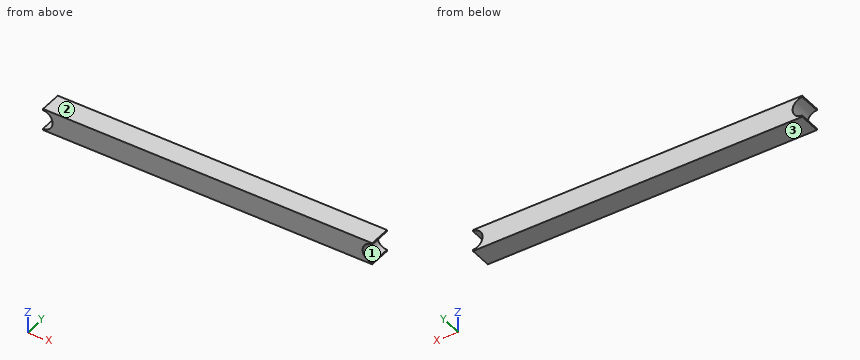
from build123d import *

# Parameters (mm, degrees)
BOX_W        = 180
BOX_H        = 12
BOX_DEPTH    = 12
POCKET_DEPTH = 12


with BuildPart() as part:
    # Box → Box (new body)
    with BuildSketch(Plane(origin=(0, -6, -6), x_dir=(1, 0, 0), z_dir=(0, 0, 1))):
        with Locations((90, 6)):
            Rectangle(BOX_W, BOX_H)
    extrude(amount=BOX_DEPTH)

    # Sketch → Pocket (cut)
    with BuildSketch(Plane(origin=(0, -6, -6), x_dir=(1, 0, 0), z_dir=(0, -1, 0))):
        with BuildLine():
            ThreePointArc((0, 0.75), (5.25, 6), (0, 11.25))
            Line((0, 11.25), (0, 0.75))
        make_face()
        with BuildLine():
            ThreePointArc((180, 11.25), (174.75, 6), (180, 0.75))
            Line((180, 11.25), (180, 0.75))
        make_face()
    extrude(amount=-POCKET_DEPTH, mode=Mode.SUBTRACT)


solid = part.part
The model under review builds one solid part; all positions refer to its coordinate system, in mm. Face numbers are marked on the shaded views. Round coordinates to 2 decimals unless told otherwise and drop trailing zeros. Loops run counter-clockwise (first coordinate to the right, second up) from the corner with the lowest first, then second, coordinate; pieces in that order, holes last. Notation, with made-up numbers: (48, 44.5) -> (107, 44.5) arc R26 cw to (107, 71.5) -> close; hole circle Ø5 at (3.25, -15). An arc over 180 degrees is marked (long way). Return JSON: item names as keys, results as strings.
(1) For line 1 (X direction, y = -5.5, z = 4.5); line 2 (X direction, y = -1, z = -0.75), list the stretches that pass through material, from the lowest coordinate up.
Solved:
{"line 1": "2.7 to 177.3", "line 2": "5.2 to 174.8"}
(2) The part is to be moulded in two halves that separate along Z. For the marked faces 1, 2 and 3, say which applies: released by +Z, released by -Z, zero draft, split by the parting line, or undercut.
Solved:
{"face 1": "undercut", "face 2": "released by +Z", "face 3": "released by -Z"}
(3) Add section A-A on y = -4.5. Write out the cut boundary in (x, z), plus the area to 3 significant figures.
Solved:
{"outline": "(0, -6) -> (180, -6) -> (180, -5.25) arc R5.25 cw to (180, 5.25) -> (180, 6) -> (0, 6) -> (0, 5.25) arc R5.25 cw to (0, -5.25) -> close", "area": "2,070 mm2"}
(4) Add section B-B on z = 0. Write out the cut boundary in (x, y).
Solved:
{"outline": "(5.25, -6) -> (174.75, -6) -> (174.75, 6) -> (5.25, 6) -> close"}
